Geometry: final body of the model. Coordinates: model frame, mm. Face numbers are marked on the shaded views. Round coordinates to 2 decimals unless told otherwise and drop trailing zeros. Order: outer loops, then holes, each group sorted by start corner. A loop starts at its lowest first (then second) coordinate and runs counter-clockwise, first axis right, second up. Notation, with made-up numbers: M 22.25,-25 L 74.25,-25 A10 ccw 74.25,-7 Z; hole C -29,-33 d4. An arc over 180 degrees is marked long. Put each result on its own line as item: value. Start each with the question number.
1) Section C-C, the plane x = -16. Return loops of the section in (y, z), then the cut area to 3 significant figures.
2) Section D-D, the plane z = 7. Return loops of the section in (x, y).
3) Material intervals for probe 1 along Z at (x, y) = (0, 68); probe 2 along X at (y, z) = (14.5, -3.5), sorted ascending. Write a range as [from, to].
4) First-contact query: P1, Ø2, axis at y = 68, z = -16, coming from the -X side; P2, Ø12, axis at x = 7.5, y = 5.5, coming from the +Z side; P3, Ø1, axis at x = -4.5, z = -26, coming from the -Y side; P4, Ø1, axis at y = 109, z = -10.5, coming from the -X side. Flat tips, straight axial feed; report the tip coordinate or a pass-through.
5) Section A-A, the plane z = 0. Return loops of the section in (x, y), then the cut area to 3 significant figures.
6) Section B-B, the plane x = -4.5. Return loops of the section in (y, z).
7) Draft query along X for the marked faces 1, 2 and 3. Return one class per face: pulls with the +X half, pulls with the -X half, needs draft (parallel to the pull), parting line crosses it, or undercut.
from build123d import *

# Parameters (mm, degrees)
SKETCH_1_R               = 27.5
EXTRUDE_1_DEPTH          = 110
EXTRUDE_1_DEPTH_BACK     = 70
SKETCH_2_R               = 26.5
CUT_EXTRUDE_1_DEPTH      = 108
CUT_EXTRUDE_1_DEPTH_BACK = 70
CUT_EXTRUDE_6_DEPTH      = 70
SKETCH_7_W               = 22
SKETCH_7_H               = 20
CUT_EXTRUDE_7_DEPTH      = 48
SKETCH_8_W               = 28
SKETCH_8_H               = 41
CUT_EXTRUDE_8_DEPTH      = 119


with BuildPart() as part:
    # 草圖1 → 填料-伸長1 (new body, two sides)
    with BuildSketch(Plane(origin=(0, 0, 0), x_dir=(1, 0, 0), z_dir=(0, 1, 0))) as extrude_1_sk:
        Circle(SKETCH_1_R)
    extrude(amount=EXTRUDE_1_DEPTH)
    extrude(extrude_1_sk.sketch, amount=-EXTRUDE_1_DEPTH_BACK)

    # 草圖2 → 除料-伸長1 (cut, two sides)
    with BuildSketch(Plane(origin=(0, 0, 0), x_dir=(1, 0, 0), z_dir=(0, 1, 0))) as cut_extrude_1_sk:
        Circle(SKETCH_2_R)
    extrude(amount=CUT_EXTRUDE_1_DEPTH, mode=Mode.SUBTRACT)
    extrude(cut_extrude_1_sk.sketch, amount=-CUT_EXTRUDE_1_DEPTH_BACK, mode=Mode.SUBTRACT)

    # 草圖6 → 除料-伸長6 (cut)
    with BuildSketch(Plane(origin=(0, 0, 0), x_dir=(1, 0, 0), z_dir=(0, 1, 0))):
        with BuildLine():
            Line((-26.5, 0), (26.300758937, 0))
            Line((26.300758937, 0), (26.5, 0))
            ThreePointArc((26.5, 0), (24.766835815, 9.426231681), (19.794049532, 17.619466595))
            Line((19.794049532, 17.619466595), (20.446397381, 18.390074337))
            ThreePointArc((20.446397381, 18.390074337), (25.676116607, 9.848199633), (27.5, 0))
            ThreePointArc((27.5, 0), (0, -27.5), (-27.5, 0))
            ThreePointArc((-27.5, 0), (-25.676116607, 9.848199633), (-20.446397381, 18.390074337))
            Line((-20.446397381, 18.390074337), (-19.794049532, 17.619466595))
            ThreePointArc((-19.794049532, 17.619466595), (-24.766835815, 9.426231681), (-26.5, 0))
        make_face()
    extrude(amount=-CUT_EXTRUDE_6_DEPTH, mode=Mode.SUBTRACT)

    # 草圖7 → 除料-伸長7 (cut)
    with BuildSketch(Plane(origin=(0, -10, 0), x_dir=(1, 0, 0), z_dir=(0, 1, 0))):
        with Locations((0, 27.910624132)):
            Rectangle(SKETCH_7_W, SKETCH_7_H)
    extrude(amount=-CUT_EXTRUDE_7_DEPTH, mode=Mode.SUBTRACT)

    # 草圖8 → 除料-伸長8 (cut)
    with BuildSketch(Plane(origin=(0, 0, 0), x_dir=(1, 0, 0), z_dir=(0, 1, 0))):
        with Locations((0, 0.320473431)):
            Rectangle(SKETCH_8_W, SKETCH_8_H)
    extrude(amount=CUT_EXTRUDE_8_DEPTH, mode=Mode.SUBTRACT)


solid = part.part
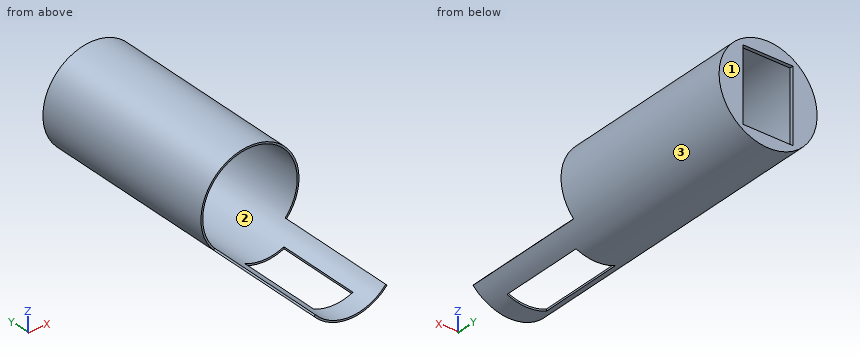
Result sheet:
1. outline: M -70,-22.37 L 110,-22.37 L 110,22.37 L 0,22.37 L 0,21.12 L 108,21.12 L 108,-21.12 L -70,-21.12 Z
1. area: 445 mm2
2. outline: M -26.59,0 L -25.56,0 L -25.56,108 L -14,108 L -14,110 L -26.59,110 Z; M 14,108 L 25.56,108 L 25.56,0 L 26.59,0 L 26.59,110 L 14,110 Z
3. probe 1: z = [-27.5, -26.5], [26.5, 27.5]
3. probe 2: x = [-27.28, -26.27], [26.27, 27.28]
4. P1: stops at x = -23.05
4. P2: stops at z = 27.46
4. P3: stops at y = -70
4. P4: stops at x = -25.62
5. outline: M -27.5,0 L -26.5,0 L -26.5,108 L -14,108 L -14,110 L -27.5,110 Z; M 14,108 L 26.5,108 L 26.5,0 L 27.5,0 L 27.5,110 L 14,110 Z
5. area: 270 mm2
6. outline: M -70,-27.13 L -58,-27.13 L -58,-26.12 L -70,-26.12 Z; M -10,-27.13 L 110,-27.13 L 110,-20.82 L 108,-20.82 L 108,-26.12 L -10,-26.12 Z; M 0,26.12 L 108,26.12 L 108,20.18 L 110,20.18 L 110,27.13 L 0,27.13 Z
7. face 1: needs draft
7. face 2: undercut
7. face 3: parting line crosses it
